Autodesk Inventor part; units mm, degrees
ref_plane "YZ Plane" through (0, 0, 0) normal (1, 0, 0) x (0, 1, 0)
ref_plane "XZ Plane" through (0, 0, 0) normal (0, 1, 0) x (-1, 0, 0)
ref_plane "XY Plane" through (0, 0, 0) normal (0, 0, 1) x (1, 0, 0)
sketch "Sketch1" plane through (0, 0, 0) normal (1, 0, 0) x (0, 1, 0)
  line L0 (-26.9875, -26.9875) -> (26.9875, -26.9875)
  line L1 (26.9875, -26.9875) -> (26.9875, 26.9875)
  line L2 (26.9875, 26.9875) -> (-26.9875, 26.9875)
  line L3 (-26.9875, 26.9875) -> (-26.9875, -26.9875)
  line L4 (-26.9875, -26.9875) -> (26.9875, 26.9875) construction
  line L5 (26.9875, -26.9875) -> (-26.9875, 26.9875) construction
  line L6 (-26, -26) -> (26, -26)
  line L7 (26, -26) -> (26, 26)
  line L8 (26, 26) -> (-26, 26)
  line L9 (-26, 26) -> (-26, -26)
  line L10 (-26, -26) -> (26, 26) construction
  line L11 (26, -26) -> (-26, 26) construction
  line L12 (-28.575, -28.575) -> (28.575, -28.575)
  line L13 (28.575, -28.575) -> (28.575, 28.575)
  line L14 (28.575, 28.575) -> (-28.575, 28.575)
  line L15 (-28.575, 28.575) -> (-28.575, -28.575)
  line L16 (-28.575, -28.575) -> (28.575, 28.575) construction
  line L17 (28.575, -28.575) -> (-28.575, 28.575) construction
  point P0 (0, 0)
  dimension "d0" = 53.975
  dimension "d1" = 53.975
  dimension "d2" = 52
  dimension "d3" = 52
  dimension "d4" = 1.5875
  dimension "d5" = 1.5875
extrude "Extrusion1" add sketch "Sketch1" along normal blind 3.175 contours L3 L2 L1 L0 | L15 L14 L13 L12
fillet "Fillet1" radius 1.0583 16 edges at (3.175, 0, 28.575) (3.175, 0, 26) (0, 0, 28.575) (3.175, 28.575, 0) (3.175, 26, 0) (3.175, -26, 0) (0, -26, 0) (3.175, -28.575, 0) (0, -28.575, 0) (3.175, 0, -26) (0, 0, -26) (3.175, 0, -28.575) (0, 28.575, 0) (0, 0, -28.575) (0, 0, 26) (0, 26, 0)
fillet "Fillet2" radius 3.175 12 edges at (2.865, 28.265, 28.265) (0.31, 28.265, 28.265) (1.5875, 28.575, 28.575) (2.865, 28.265, -28.265) (0.31, 28.265, -28.265) (1.5875, 28.575, -28.575) (1.5875, -28.575, -28.575) (0.31, -28.265, -28.265) (2.865, -28.265, -28.265) (2.865, -28.265, 28.265) (0.31, -28.265, 28.265) (1.5875, -28.575, 28.575)
equation "\"d0\" = sensorHolderSensorWidth"
equation "\"d1\" = sensorHolderSensorHeight"
equation "\"d2\" = detectorWidth"
equation "\"d3\" = detectorHeight"
equation "\"d4\" = 0.5 * oRingWidth"
equation "\"d5\" = 0.5 * oRingWidth"
equation "\"d6\" = sensorHolderORing"
equation "\"d8\" = 0.333333 * oRingWidth"
equation "\"d9\" = oRingWidth"
equation "\"acrylicThickness\" = 6.35"
equation "\"height\" = 101.6"
equation "\"width\" = 101.6"
equation "\"depth\" = 101.6"
equation "\"mirrorAngle\" = 5deg"
equation "\"detectorWidth\" = 52"
equation "\"detectorHeight\" = 52"
equation "\"mirrorThickness\" = 3"
equation "\"fresnelThickness\" = 0.1"
equation "\"focalLength\" = 76.2"
equation "\"ior\" = 1.49"
equation "\"centerThickness\" = 1.524"
equation "\"fresnelAngle\" = 90deg"
equation "\"fresnelEffectiveDiameter\" = 76.2"
equation "\"mirrorSuppourtWidth\" = 38.1"
equation "\"backGrooveBit\" = 4.8006"
equation "\"sensorHolderWidth\" = 88.9"
equation "\"sensorHolderHeight\" = 88.9"
equation "\"sensorHolderSensorHeight\" = 53.975"
equation "\"sensorHolderSensorWidth\" = 53.975"
equation "\"sensorHolderORingGroove\" = 3.175"
equation "\"sensorHolderORing\" = 3.175"
equation "\"sensorHolderFlushORing\" = 3.175"
equation "\"sensorHolderFlushORingID\" = 304.8"
equation "\"sensorHolderORingID\" = 203.2"
equation "\"oRingWidth\" = 3.175"
equation "\"frontBackORingID\" = 419.1"
equation "\"topBottomHorizontalMirrorGroove\" = 12.7"
equation "\"backMirrorGroove\" = 6.35"
equation "\"mirrorGroove\" = 19.05"
equation "\"mirrorGrooveFillet\" = 6.35"
equation "\"fresnelChamfer\" = 6.35"
equation "\"mirrorGrooveDrill\" = 6.35"
equation "\"mirrorGrooveMill\" = 3.175"
equation "\"fresnelMirrorChamfer\" = 6.35"
equation "\"detectorOpeningWidth\" = 76.2"
equation "\"detectorOpeningHeight\" = 76.2"
properties part number "sensorORing" material "Rubber"
CAD build for the part. Positions are in the model's coordinates, mm. Round coordinates to 2 decimals unless told otherwise and drop trailing zeros. Order: outer loops, then holes, each group sorted by start corner. A loop starts at its lowest first (then second) coordinate and runs counter-clockwise, first axis right, second up. Notation, with made-up numbers: (65.25, 26) -> (70.25, 26) arc R23 ccw to (70.25, 51) -> close; hole circle Ø6 at (53.25, -16). An arc over 180 degrees is marked (long way). Write item = value, one per line. Start each with the question number.
(1) Probe line 1 (Y direction, x = 1.35, z = -16.5) (3 decimals); line 2 (Z direction, x = 3.05, y = 16). List the from-to ranges inside material, lowest first. Write a range as [from, to].
(2) Cut at C-C, the plane x = 0.5. List the corners of the cut face in (y, z), then the cut area to 3 significant figures.
(3) Cut at A-A, the plane y = 19.5. List the corners of the cut face in (x, z) (3 decimals), then the cut area to 3 significant figures.
Model answer:
q1.line_1 = [-28.575, -26], [26, 28.575]
q1.line_2 = [-28.02, -26.56], [26.56, 28.02]
q2.outline = (-28.42, -25.4) arc R3.02 ccw to (-25.4, -28.42) -> (25.4, -28.42) arc R3.02 ccw to (28.42, -25.4) -> (28.42, 25.4) arc R3.02 ccw to (25.4, 28.42) -> (-25.4, 28.42) arc R3.02 ccw to (-28.42, 25.4) -> close; hole (-26.16, -26.16) -> (26.16, -26.16) -> (26.16, 26.16) -> (-26.16, 26.16) -> close
q2.area = 485 mm2
q3.outline = (0, -27.517) arc R1.058 ccw to (1.058, -28.575) -> (2.117, -28.575) arc R1.058 ccw to (3.175, -27.517) -> (3.175, -27.058) arc R1.058 ccw to (2.117, -26) -> (1.058, -26) arc R1.058 ccw to (0, -27.058) -> close; (0, 27.058) arc R1.058 ccw to (1.058, 26) -> (2.117, 26) arc R1.058 ccw to (3.175, 27.058) -> (3.175, 27.517) arc R1.058 ccw to (2.117, 28.575) -> (1.058, 28.575) arc R1.058 ccw to (0, 27.517) -> close
q3.area = 14.4 mm2
